```python
from build123d import *

# Parameters (mm, degrees)
SKETCH3_W          = 20.8
SKETCH3_H          = 20.8
CUT_EXTRUDE1_DEPTH = 20
CUT_EXTRUDE2_DEPTH = 65.031242546
CUT_EXTRUDE5_START = 14
CUT_EXTRUDE5_DEPTH = 51.031242546
SKETCH5_R          = 1.75
CUT_EXTRUDE6_DEPTH = 65.031242546
CUT_EXTRUDE7_START = 3
SKETCH5_3_R        = 4.5
SKETCH5_3_R_2      = 1.75
CUT_EXTRUDE7_DEPTH = 62.031242546
CIRPATTERN1_COUNT  = 4


with BuildPart() as part:
    # Sketch2 → Loft1 section 0
    with BuildSketch(Plane(origin=(0, 30, 0), x_dir=(1, 0, 0), z_dir=(0, 1, 0))):
        with BuildLine():
            Line((12.5, -12.5), (-12.5, -12.5))
            Line((-12.5, -12.5), (-12.5, 12.5))
            Line((-12.5, 12.5), (12.5, 12.5))
            Line((12.5, 12.5), (12.5, -12.5))
        make_face()
    # Sketch1 → Loft1 section 1
    with BuildSketch(Plane(origin=(0, 0, 0), x_dir=(1, 0, 0), z_dir=(0, 1, 0))):
        with BuildLine():
            Line((40, -40), (-40, -40))
            Line((-40, -40), (-40, 40))
            Line((-40, 40), (40, 40))
            Line((40, 40), (40, -40))
        make_face()
    loft()

    # Sketch3 → Cut-Extrude1 (cut)
    with BuildSketch(Plane(origin=(0, 30, 0), x_dir=(1, 0, 0), z_dir=(0, 1, 0))):
        Rectangle(SKETCH3_W, SKETCH3_H)
    extrude(amount=-CUT_EXTRUDE1_DEPTH, mode=Mode.SUBTRACT)

    # Sketch4 → Cut-Extrude2 (cut, through all)
    with BuildSketch(Plane.XY):
        with BuildLine():
            ThreePointArc((1.75, 20), (1.237436867, 21.237436867), (0, 21.75))
            Line((0, 21.75), (0, 18.25))
            ThreePointArc((0, 18.25), (1.237436867, 18.762563133), (1.75, 20))
        make_face()
        with BuildLine():
            Line((0, 18.25), (0, 21.75))
            ThreePointArc((0, 21.75), (-1.75, 20), (0, 18.25))
        make_face()
    extrude(amount=CUT_EXTRUDE2_DEPTH, mode=Mode.SUBTRACT)

    # Sketch4_3 → Cut-Extrude5 (cut, through all)
    with BuildSketch(Plane.XY.offset(CUT_EXTRUDE5_START)):
        with BuildLine():
            ThreePointArc((4.5, 20), (3.181980515, 23.181980515), (0, 24.5))
            Line((0, 24.5), (0, 21.75))
            ThreePointArc((0, 21.75), (1.237436867, 21.237436867), (1.75, 20))
            ThreePointArc((1.75, 20), (1.237436867, 18.762563133), (0, 18.25))
            Line((0, 18.25), (0, 15.5))
            ThreePointArc((0, 15.5), (3.181980515, 16.818019485), (4.5, 20))
        make_face()
        with BuildLine():
            Line((0, 21.75), (0, 24.5))
            ThreePointArc((0, 24.5), (-4.5, 20), (0, 15.5))
            Line((0, 15.5), (0, 18.25))
            ThreePointArc((0, 18.25), (-1.75, 20), (0, 21.75))
        make_face()
    extrude(amount=CUT_EXTRUDE5_DEPTH, mode=Mode.SUBTRACT)

    # Sketch5 → Cut-Extrude6 (cut, through all)
    with BuildSketch(Plane(origin=(0, 0, 0), x_dir=(1, 0, 0), z_dir=(0, 1, 0))):
        with Locations(Location((-31.514718626, 31.514718626, 0), (0, 0, 135))):
            Circle(SKETCH5_R)
    cut_extrude6 = extrude(amount=CUT_EXTRUDE6_DEPTH, mode=Mode.SUBTRACT)

    # Sketch5_3 → Cut-Extrude7 (cut, through all)
    with BuildSketch(Plane(origin=(0, 0, 0), x_dir=(1, 0, 0), z_dir=(0, 1, 0)).offset(CUT_EXTRUDE7_START)):
        with Locations(Location((-31.514718626, 31.514718626, 0), (0, 0, 135))):
            Circle(SKETCH5_3_R)
        with Locations(Location((-31.514718626, 31.514718626, 0), (0, 0, 270))):
            Circle(SKETCH5_3_R_2, mode=Mode.SUBTRACT)
    cut_extrude7 = extrude(amount=CUT_EXTRUDE7_DEPTH, mode=Mode.SUBTRACT)

    # CirPattern1: Cut-Extrude6, Cut-Extrude7 ×4 about axis
    cirpattern1_axis = Axis((0, 0, 0), (0, 1, 0))
    add([cut_extrude6.rotate(cirpattern1_axis, i * 360 / CIRPATTERN1_COUNT) for i in range(1, CIRPATTERN1_COUNT)], mode=Mode.SUBTRACT)
    add([cut_extrude7.rotate(cirpattern1_axis, i * 360 / CIRPATTERN1_COUNT) for i in range(1, CIRPATTERN1_COUNT)], mode=Mode.SUBTRACT)


solid = part.part
```
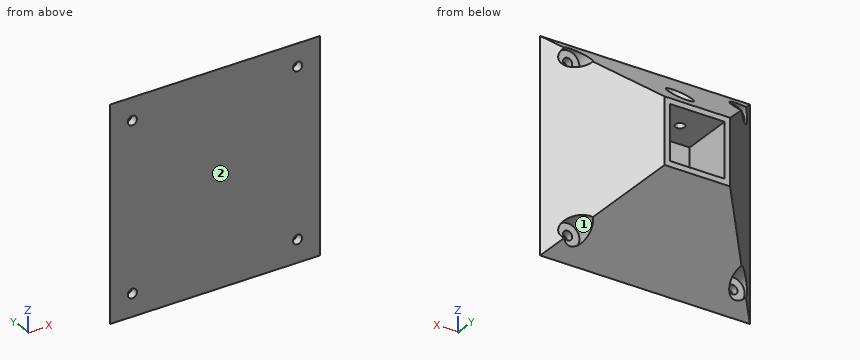
Design review of the part built by this model. Coordinates are the model's own, in mm. Face numbers are marked on the shaded views. Coordinates: 2 decimals unless noted, no trailing zeros. One line per question, with ' | ' between items.
(1) We need section A-A (y = 4). Count the separate pieces of the cut face and the enclosed holes in it, and give its area (3 significant figures).
Filled in:
separate pieces: 1 | enclosed holes: 4 | area: 5,030 mm^2
(2) Draft analysis for pull direction Z (two halves, no side actions). For the marked faces 1 and 2, state which applies: released by +Z, released by -Z, zero draft, split by the parting line, or undercut.
Filled in:
face 1: undercut | face 2: zero draft
(3) Wall thickness on probe 1 along Y at (x, z) = (10, 10); probe 2 along X at (y, z) = (19.5, -6) (3 decimals); probe 3 along Z at (x, y) = (4.5, 27.5): over which ranges is each line inside the solid? List them lowest first.
Filled in:
probe 1: y = 0 to 10 | probe 2: x = -22.125 to -10.4, 10.4 to 22.125 | probe 3: z = -14.79 to -10.4, 10.4 to 14.79
(4) For pin 1 Ø5 at (x, z) = (-28.5, 30) entering from +Y; pin 2 Ø23 at (x, z) = (-4, -4.5) entering from +Y; pin 3 Ø8 at (x, y) = (-1, 6.5) entering from -Z; pin 4 Ø8 at (x, z) = (-31.51, -31.51) entering from +Y, all flat-tipped, find the tip position at first contact; note any pin that passes through.
Filled in:
pin 1: stops at y = 13.47 | pin 2: stops at y = 30 | pin 3: stops at z = -37.71 | pin 4: stops at y = 3
